Input: part model. Units: mm. Frame: model coordinates. Coordinates: 2 decimals unless noted, no trailing zeros. Write each loop counter-clockwise with the first axis right and the second up, starting at its lowest first coordinate (ties: lowest second). Pieces come first, ordered by that corner, then holes. Notation, with made-up numbers: (1.25, 30.5) - (45.25, 30.5) arc R18 ccw to (45.25, 61.5) - close; hole circle Ø7 at (-22.5, 87). An arc over 180 degrees is marked (long way). Put each result on its own line as item: value. Start each with the question number.
1. Line query: line 1 (Z direction, x = 90, y = 0.55); line 2 (X direction, y = 0.45, z = 30); line 3 (X direction, y = 0.35, z = 28). Output: solid intervals per line, ascending.
2. Pin query (flat end, axial travel): pin 1 (2.5 mm diameter, centred on x = -90, z = 28, fed in from -Y). Return the tip coordinate at first contact, or that it passes through.
3. Cut plane B-B, the plane x = -14. Return loops of the section in (y, z).
4. Cut plane A-A, the plane y = 0.85. Count the separate pieces of the cut face and the enclosed holes in it, and give its area (3 significant figures).
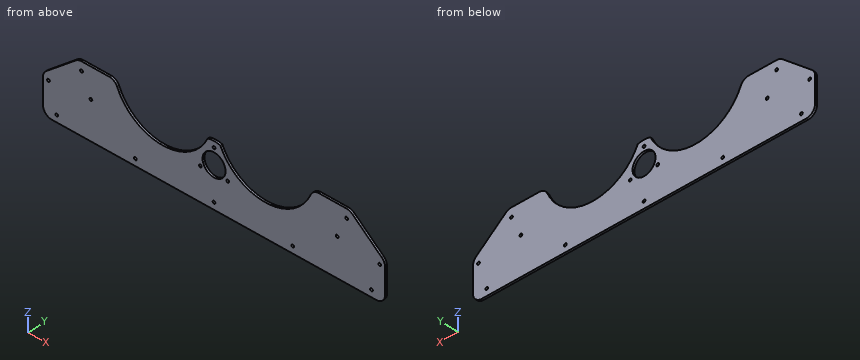
from build123d import *

# Parameters (mm, degrees)
BOSS_EXTRU_1_DEPTH      = 1.5
ESQUISSE2_R             = 1
ENL_V_MAT_EXTRU_1_DEPTH = 135.637476209
ESQUISSE4_R             = 36
ENL_V_MAT_EXTRU_3_DEPTH = 135.637476209
CONG_1_R                = 6.5
ESQUISSE3_R             = 8.4
ESQUISSE3_R_2           = 1
ENL_V_MAT_EXTRU_2_DEPTH = 1.5
ENL_V_MAT_EXTRU_4_DEPTH = 135.637476209


with BuildPart() as part:
    # Esquisse1 → Boss.-Extru.1 (new body)
    with BuildSketch(Plane(origin=(0, 0, 0), x_dir=(1, 0, 0), z_dir=(0, 1, 0))):
        Polygon((99.25, -50), (125, -28.393184497), (125, 0), (0, 0), (0, -50), align=None)
    extrude(amount=BOSS_EXTRU_1_DEPTH)

    # Esquisse2 → Enlèv. mat.-Extru.1 (cut, through all)
    with BuildSketch(Plane(origin=(0, 1.5, 0), x_dir=(1, 0, 0), z_dir=(0, 1, 0))):
        with Locations((0, -5)):
            Circle(ESQUISSE2_R)
        with Locations(Location((57.5, -5, 0), (0, 0, 270))):
            Circle(ESQUISSE2_R)
        with Locations(Location((115, -5, 0), (0, 0, 270))):
            Circle(ESQUISSE2_R)
        with Locations(Location((96.884193477, -43.5, 0), (0, 0, 270))):
            Circle(ESQUISSE2_R)
        with Locations(Location((90, -28, 0), (0, 0, 270))):
            Circle(ESQUISSE2_R)
        with Locations(Location((121, -25, 0), (0, 0, 270))):
            Circle(ESQUISSE2_R)
    extrude(amount=-ENL_V_MAT_EXTRU_1_DEPTH, mode=Mode.SUBTRACT)

    # Esquisse4 → Enlèv. mat.-Extru.3 (cut, through all)
    with BuildSketch(Plane(origin=(0, 1.5, 0), x_dir=(1, 0, 0), z_dir=(0, 1, 0))):
        with Locations((37.5, -60)):
            Circle(ESQUISSE4_R)
    extrude(amount=-ENL_V_MAT_EXTRU_3_DEPTH, mode=Mode.SUBTRACT)

    # Congé1
    cong_1_edges = [part.edges().sort_by_distance(p)[0] for p in [
        (125, 0.75, 28.393184497),
        (99.25, 0.75, 50),
        (125, 0.75, 0),
        (72.083232932, 0.75, 50),
    ]]
    fillet(cong_1_edges, radius=CONG_1_R)

    # Symétrie1: part across plane


with BuildPart() as part_1:
    add(part.part)
    add(part.part.mirror(Plane(origin=(0, 0, 0), x_dir=(0, 0, 1), z_dir=(1, 0, 0))))

    # Esquisse3 → Enlèv. mat.-Extru.2 (cut)
    with BuildSketch(Plane(origin=(0, 1.5, 0), x_dir=(1, 0, 0), z_dir=(0, 1, 0))):
        with Locations(Location((0, -30, 0), (0, 0, 270))):
            Circle(ESQUISSE3_R)
        with Locations(Location((0, -41.547005384, 0), (0, 0, 270))):
            Circle(ESQUISSE3_R_2)
        with Locations(Location((-10, -24.226497308, 0), (0, 0, 270))):
            Circle(ESQUISSE3_R_2)
        with Locations(Location((10, -24.226497308, 0), (0, 0, 270))):
            Circle(ESQUISSE3_R_2)
    extrude(amount=-ENL_V_MAT_EXTRU_2_DEPTH, mode=Mode.SUBTRACT)

    # Esquisse5 → Enlèv. mat.-Extru.4 (cut, through all)
    with BuildSketch(Plane(origin=(0, 1.5, 0), x_dir=(1, 0, 0), z_dir=(0, 1, 0))):
        with BuildLine():
            Line((7.702133216, -44.02416286), (7.702133216, -51.975452854))
            Line((7.702133216, -51.975452854), (-8.276969641, -51.975452854))
            Line((-8.276969641, -51.975452854), (-6.500509259, -44.619965095))
            ThreePointArc((-6.500509259, -44.619965095), (0.670611742, -45.985940069), (7.702133216, -44.02416286))
        make_face()
    extrude(amount=-ENL_V_MAT_EXTRU_4_DEPTH, mode=Mode.SUBTRACT)


solid = part_1.part
Report:
1. line 1: z = 0 to 27, 29 to 50
1. line 2: x = -123.05 to -57.4, -17.6 to -8.4, 8.4 to 17.6, 57.4 to 123.05
1. line 3: x = -124.44 to -91, -89 to -53.99, -21.01 to -8.16, 8.16 to 21.01, 53.99 to 89, 91 to 124.44
2. pin 1: stops at y = 0
3. outline: (0, 0) - (1.5, 0) - (1.5, 32.73) - (0, 32.73) - close
4. separate pieces: 1
4. enclosed holes: 15
4. area: 8,970 mm^2
